Read the model definition and answer for the solid it produces. Units are mm, in the model's axes. Face numbers are marked on the shaded views. Give positions to 0.01 mm unless a question says otherwise; leave off trailing zeros. Loops run counter-clockwise (first coordinate to the right, second up) from the corner with the lowest first, then second, coordinate; pieces in that order, holes last.
(1) Straight lines are drawn through the part: probe 1 along Z at (x, y) = (6.5, 3); probe 2 along X at (y, z) = (3.75, 5.5); probe 3 along Y at (x, z) = (-25, -8). For each, find the intervals that lie inside material, in ascending order.
(2) Determine the mould class of the marked faces 1, 2 and 3 for opening direction X: pulls with the +X half, pulls with the -X half, needs draft (parallel to the pull), parting line crosses it, or undercut.
(3) Find section B-B, the plane z = 11. Write down the section's boundary in (x, y), then the cut area to 3 significant figures.
(4) Find section C-C, the plane y = 6.25. Write down the section's boundary in (x, z), then the cut area to 3 significant figures.
(5) Find section A-A, the plane x = -15. Write down the section's boundary in (y, z).
(6) Each of these flat-tipped pins is pushed along its axis until it touches: P1, Ø1.2, axis at x = -8, y = 3, coming from the +Z side; P2, Ø1.5, axis at x = 18, z = -13.5, coming from the +Y side; P3, Ø0.8, axis at y = 3, z = -18, coming from the -X side. Where does it stop, or does it pass through?
```python
from build123d import *

# Parameters (mm, degrees)
SKETCH_1_W          = 65
SKETCH_1_H          = 45
EXTRUDE_1_DEPTH     = 2
SKETCH_2_W          = 59.7
SKETCH_2_H          = 39.7
EXTRUDE_2_DEPTH     = 2.5
EXTRUDE_3_DEPTH     = 5.8
SKETCH_4_W          = 0.15
SKETCH_4_H          = 32
CUT_EXTRUDE_1_DEPTH = 3.3
SKETCH_5_W          = 54.7
SKETCH_5_H          = 34.7
CUT_EXTRUDE_2_DEPTH = 2.5


with BuildPart() as part:
    # 草图1 → 凸台-拉伸1 (new body)
    with BuildSketch(Plane(origin=(0, 0, 0), x_dir=(1, 0, 0), z_dir=(0, 1, 0))):
        Rectangle(SKETCH_1_W, SKETCH_1_H)
    extrude(amount=EXTRUDE_1_DEPTH)

    # 草图2 → 凸台-拉伸2 (add)
    with BuildSketch(Plane(origin=(0, 2, 0), x_dir=(1, 0, 0), z_dir=(0, 1, 0))):
        Rectangle(SKETCH_2_W, SKETCH_2_H)
    extrude(amount=EXTRUDE_2_DEPTH)

    # 草图3 → 凸台-拉伸3 (add)
    with BuildSketch(Plane(origin=(0, 2, 0), x_dir=(1, 0, 0), z_dir=(0, 1, 0))):
        Polygon((-30, -16), (-29.85, -16), (-29.85, 16), (-30, 16), (-31.25, 17.25), (-32.5, 16), (-32.5, -16), (-31.25, -17.25), align=None)
    extrude(amount=EXTRUDE_3_DEPTH)

    # 草图4 → 切除-拉伸1 (cut)
    with BuildSketch(Plane(origin=(0, 7.8, 0), x_dir=(1, 0, 0), z_dir=(0, 1, 0))):
        with Locations((-29.925, 0)):
            Rectangle(SKETCH_4_W, SKETCH_4_H)
    extrude(amount=-CUT_EXTRUDE_1_DEPTH, mode=Mode.SUBTRACT)

    # 草图5 → 切除-拉伸2 (cut)
    with BuildSketch(Plane(origin=(0, 4.5, 0), x_dir=(1, 0, 0), z_dir=(0, 1, 0))):
        Rectangle(SKETCH_5_W, SKETCH_5_H)
    extrude(amount=-CUT_EXTRUDE_2_DEPTH, mode=Mode.SUBTRACT)


solid = part.part
```
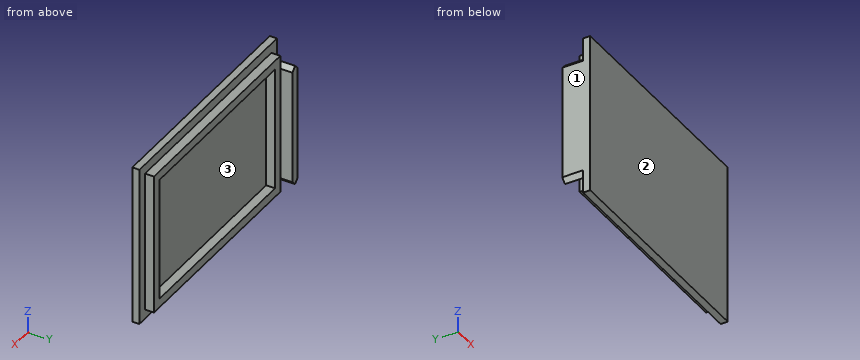
Entries:
1. probe 1: z = -19.85 to -17.35, 17.35 to 19.85
1. probe 2: x = -32.5 to -27.35, 27.35 to 29.85
1. probe 3: y = 0 to 2
2. face 1: pulls with the -X half
2. face 2: needs draft
2. face 3: undercut
3. outline: (-32.5, 0) - (32.5, 0) - (32.5, 2) - (29.85, 2) - (29.85, 4.5) - (27.35, 4.5) - (27.35, 2) - (-27.35, 2) - (-27.35, 4.5) - (-30, 4.5) - (-30, 7.8) - (-32.5, 7.8) - close
3. area: 157 mm2
4. outline: (-32.5, -16) - (-31.25, -17.25) - (-30, -16) - (-30, 16) - (-31.25, 17.25) - (-32.5, 16) - close
4. area: 83.1 mm2
5. outline: (0, -22.5) - (2, -22.5) - (2, -19.85) - (4.5, -19.85) - (4.5, -17.35) - (2, -17.35) - (2, 17.35) - (4.5, 17.35) - (4.5, 19.85) - (2, 19.85) - (2, 22.5) - (0, 22.5) - close
6. P1: stops at z = 19.85
6. P2: stops at y = 2
6. P3: stops at x = -29.85
